```python
from build123d import *

# Parameters (mm, degrees)
PAD_DEPTH    = 14
SKETCH001_R  = 1.7
POCKET_DEPTH = 8.001


with BuildPart() as part:
    # Sketch → Pad (new body)
    with BuildSketch(Plane.XY):
        with BuildLine():
            Line((-12.5, 0), (12.5, 0))
            Line((12.5, 0), (12.5, 8))
            Line((12.5, 8), (11.2, 8))
            Line((11.2, 8), (10.038893, 5.947726))
            ThreePointArc((10.038893, 5.947726), (10.04085, 5.648867), (10.3, 5.5))
            Line((10.3, 5.5), (11, 5.5))
            Line((11, 5.5), (11, 2))
            Line((11, 2), (-11, 2))
            Line((-11, 2), (-11, 5.5))
            Line((-11, 5.5), (-10.3, 5.5))
            ThreePointArc((-10.3, 5.5), (-10.04085, 5.648867), (-10.038893, 5.947726))
            Line((-10.038893, 5.947726), (-11.2, 8))
            Line((-11.2, 8), (-12.5, 8))
            Line((-12.5, 8), (-12.5, 0))
        make_face()
    extrude(amount=PAD_DEPTH)

    # Sketch001 → Pocket (cut, through all)
    with BuildSketch(Plane.XZ):
        with Locations((0, 7)):
            Circle(SKETCH001_R)
    extrude(amount=-POCKET_DEPTH, mode=Mode.SUBTRACT)


solid = part.part
```
Here's how the part is built. I have some questions about the finished solid (model axes, mm). A direction names the side the tool comes from. Round coordinates to 2 decimals unless told otherwise and drop trailing zeros. Order: outer loops, then holes, each group sorted by start corner. A loop starts at its lowest first (then second) coordinate and runs counter-clockwise, first axis right, second up. Notation, with made-up numbers: M -35.75,25 L -21.75,25 A26 ccw -21.75,45 Z; hole C 40.5,5 d4. An arc over 180 degrees is marked long. Answer as CSV lines item,"result".
Item 1: We'd pull the mould along X, two halves only. Please class faces 4 (the flat face through (-11, 4, 7)), 5 (the flat face through (12, 8, 7)), 6 (the flat face through (-12.5, 4, 7)): +X half, -X half, draft (parallel to the pull), parting line (faces both ways), or undercut.
From the geometry:
face 4,"undercut"
face 5,"draft"
face 6,"-X half"
Item 2: Please list where these lines run through material, in increasing order: L1, parallel to X at y = 3.5, z = 11; L2, parallel to Z at x = 0, y = 1.3; L3, parallel to Y at x = 0.5, z = 12. Write a range as [from, to].
From the geometry:
L1,"[-12.5, -11], [11, 12.5]"
L2,"[0, 5.3], [8.7, 14]"
L3,"[0, 2]"
Item 3: Imagine slicing it at C-C on x = 0. List the corners of the cut face in (y, z) for me.
From the geometry:
outline,"M 0,0 L 2,0 L 2,5.3 L 0,5.3 Z; M 0,8.7 L 2,8.7 L 2,14 L 0,14 Z"
Item 4: Which directions (+Z, -Z, +X, -X, +Y, -Y) give clear straight access to the entire face, cutting with the end or side of a thin tool? Please do faces 1 (the flat face through (11, 4, 7)), 2 (the flat face through (-10.61, 6.96, 6.9)), 3 (the flat face through (-3, 0, 7)).
From the geometry:
face 1,"+Z, -Z"
face 2,"+Z, -Z, +Y"
face 3,"+Z, -Z, +X, -X, -Y"
Item 5: Imagine slicing it at A-A on z = 7. List the corners of the cut face in (x, y) for me.
From the geometry:
outline,"M -12.5,0 L -1.7,0 L -1.7,2 L -11,2 L -11,5.5 L -10.3,5.5 A0.3 ccw -10.04,5.95 L -11.2,8 L -12.5,8 Z; M 1.7,0 L 12.5,0 L 12.5,8 L 11.2,8 L 10.04,5.95 A0.3 ccw 10.3,5.5 L 11,5.5 L 11,2 L 1.7,2 Z"
Item 6: For pin 1 (4.5 mm diameter, centred on x = 0, z = 7, fed in from +Y), with a flat end and sliding along its axis, tell me the tip position at first contact or that it passes through.
From the geometry:
pin 1,"y = 2"
Item 7: Imagine slicing it at B-B on y = 5. List the corners of the cut face in (x, z) for me.
From the geometry:
outline,"M -12.5,0 L -11,0 L -11,14 L -12.5,14 Z; M 11,0 L 12.5,0 L 12.5,14 L 11,14 Z"
Item 8: Imagine slicing it at D-D on z = 9.5. List the corners of the cut face in (x, y) for me, and give its area (3 significant figures).
From the geometry:
outline,"M -12.5,0 L 12.5,0 L 12.5,8 L 11.2,8 L 10.04,5.95 A0.3 ccw 10.3,5.5 L 11,5.5 L 11,2 L -11,2 L -11,5.5 L -10.3,5.5 A0.3 ccw -10.04,5.95 L -11.2,8 L -12.5,8 Z"
area,"70.4 mm2"
